For this review, take the finished solid that the model builds, in its own axes (mm). Round coordinates to 2 decimals unless told otherwise and drop trailing zeros. One line per question, with ' | ' between items. Start each with the question number.
1) Mouldability with a two-part tool opening along Y and no side actions: class faces 1 (the face through (-34.375, 0, 1)), 2 (the face through (-10.09, 26.51, 1.23)) as pulls with the +Y half, pulls with the -Y half, needs draft (parallel to the pull), parting line crosses it, or undercut.
2) We need section A-A (x = 0.5). State how many separate pieces and enclosed holes the cut face has, and give its area (3 significant figures).
3) For pin 1 Ø4 at (x, y) = (-19.875, -35.125) entering from +Z; pin 2 Ø2 at (x, y) = (-9.875, -15.125) entering from -Z, all flat-tipped, find the tip position at first contact; note any pin that passes through.
```python
from build123d import *

# Parameters (mm, degrees)
F0_W     = 68.75
F0_H     = 78.75
F0_R     = 1.65
F1_DEPTH = 2.5
F2_R     = 4.5


with BuildPart() as f1:
    # F0 (on Top) → F1 (new body)
    with BuildSketch(Plane.XY):
        Rectangle(F0_W, F0_H)
        with Locations((-29.875, -35.125)):
            Circle(F0_R, mode=Mode.SUBTRACT)
        with Locations((-19.875, -35.125)):
            Circle(F0_R, mode=Mode.SUBTRACT)
        with Locations((-29.875, -25.125)):
            Circle(F0_R, mode=Mode.SUBTRACT)
        with Locations((-19.875, -25.125)):
            Circle(F0_R, mode=Mode.SUBTRACT)
        with Locations((-9.875, -35.125)):
            Circle(F0_R, mode=Mode.SUBTRACT)
        with Locations((-9.875, -25.125)):
            Circle(F0_R, mode=Mode.SUBTRACT)
        with Locations((-29.875, -15.125)):
            Circle(F0_R, mode=Mode.SUBTRACT)
        with Locations((-19.875, -15.125)):
            Circle(F0_R, mode=Mode.SUBTRACT)
        with Locations((-29.875, -5.125)):
            Circle(F0_R, mode=Mode.SUBTRACT)
        with Locations((-19.875, -5.125)):
            Circle(F0_R, mode=Mode.SUBTRACT)
        with Locations((-9.875, -15.125)):
            Circle(F0_R, mode=Mode.SUBTRACT)
        with Locations((-9.875, -5.125)):
            Circle(F0_R, mode=Mode.SUBTRACT)
        with Locations((0.125, -35.125)):
            Circle(F0_R, mode=Mode.SUBTRACT)
        with Locations((10.125, -35.125)):
            Circle(F0_R, mode=Mode.SUBTRACT)
        with Locations((0.125, -25.125)):
            Circle(F0_R, mode=Mode.SUBTRACT)
        with Locations((10.125, -25.125)):
            Circle(F0_R, mode=Mode.SUBTRACT)
        with Locations((20.125, -35.125)):
            Circle(F0_R, mode=Mode.SUBTRACT)
        with Locations((30.125, -35.125)):
            Circle(F0_R, mode=Mode.SUBTRACT)
        with Locations((20.125, -25.125)):
            Circle(F0_R, mode=Mode.SUBTRACT)
        with Locations((30.125, -25.125)):
            Circle(F0_R, mode=Mode.SUBTRACT)
        with Locations((0.125, -15.125)):
            Circle(F0_R, mode=Mode.SUBTRACT)
        with Locations((10.125, -15.125)):
            Circle(F0_R, mode=Mode.SUBTRACT)
        with Locations((0.125, -5.125)):
            Circle(F0_R, mode=Mode.SUBTRACT)
        with Locations((10.125, -5.125)):
            Circle(F0_R, mode=Mode.SUBTRACT)
        with Locations((20.125, -15.125)):
            Circle(F0_R, mode=Mode.SUBTRACT)
        with Locations((30.125, -15.125)):
            Circle(F0_R, mode=Mode.SUBTRACT)
        with Locations((20.125, -5.125)):
            Circle(F0_R, mode=Mode.SUBTRACT)
        with Locations((30.125, -5.125)):
            Circle(F0_R, mode=Mode.SUBTRACT)
        with Locations((-29.875, 4.875)):
            Circle(F0_R, mode=Mode.SUBTRACT)
        with Locations((-19.875, 4.875)):
            Circle(F0_R, mode=Mode.SUBTRACT)
        with Locations((-29.875, 14.875)):
            Circle(F0_R, mode=Mode.SUBTRACT)
        with Locations((-19.875, 14.875)):
            Circle(F0_R, mode=Mode.SUBTRACT)
        with Locations((-9.875, 4.875)):
            Circle(F0_R, mode=Mode.SUBTRACT)
        with Locations((-9.875, 14.875)):
            Circle(F0_R, mode=Mode.SUBTRACT)
        with Locations((-29.875, 24.875)):
            Circle(F0_R, mode=Mode.SUBTRACT)
        with Locations((-19.875, 24.875)):
            Circle(F0_R, mode=Mode.SUBTRACT)
        with Locations((-29.875, 34.875)):
            Circle(F0_R, mode=Mode.SUBTRACT)
        with Locations((-19.875, 34.875)):
            Circle(F0_R, mode=Mode.SUBTRACT)
        with Locations((-9.875, 24.875)):
            Circle(F0_R, mode=Mode.SUBTRACT)
        with Locations((-9.875, 34.875)):
            Circle(F0_R, mode=Mode.SUBTRACT)
        with Locations((0.125, 4.875)):
            Circle(F0_R, mode=Mode.SUBTRACT)
        with Locations((10.125, 4.875)):
            Circle(F0_R, mode=Mode.SUBTRACT)
        with Locations((0.125, 14.875)):
            Circle(F0_R, mode=Mode.SUBTRACT)
        with Locations((10.125, 14.875)):
            Circle(F0_R, mode=Mode.SUBTRACT)
        with Locations((20.125, 4.875)):
            Circle(F0_R, mode=Mode.SUBTRACT)
        with Locations((30.125, 4.875)):
            Circle(F0_R, mode=Mode.SUBTRACT)
        with Locations((20.125, 14.875)):
            Circle(F0_R, mode=Mode.SUBTRACT)
        with Locations((30.125, 14.875)):
            Circle(F0_R, mode=Mode.SUBTRACT)
        with Locations((0.125, 24.875)):
            Circle(F0_R, mode=Mode.SUBTRACT)
        with Locations((10.125, 24.875)):
            Circle(F0_R, mode=Mode.SUBTRACT)
        with Locations((0.125, 34.875)):
            Circle(F0_R, mode=Mode.SUBTRACT)
        with Locations((10.125, 34.875)):
            Circle(F0_R, mode=Mode.SUBTRACT)
        with Locations((20.125, 24.875)):
            Circle(F0_R, mode=Mode.SUBTRACT)
        with Locations((30.125, 24.875)):
            Circle(F0_R, mode=Mode.SUBTRACT)
        with Locations((20.125, 34.875)):
            Circle(F0_R, mode=Mode.SUBTRACT)
        with Locations((30.125, 34.875)):
            Circle(F0_R, mode=Mode.SUBTRACT)
    extrude(amount=F1_DEPTH)

    # F2
    f2_edges = [f1.edges().sort_by_distance(p)[0] for p in [
        (34.375, 39.375, 1.25),
        (34.375, -39.375, 1.25),
        (-34.375, 39.375, 1.25),
        (-34.375, -39.375, 1.25),
    ]]
    fillet(f2_edges, radius=F2_R)


solid = f1.part
```
Answers below:
1) face 1: needs draft | face 2: undercut
2) separate pieces: 9 | enclosed holes: 0 | area: 133 mm^2
3) pin 1: z = 2.5 | pin 2: through
